Work out the finished part from the listing and answer in its coordinate system (mm). Face numbers are marked on the shaded views. A direction names the side the tool comes from. Round coordinates to 2 decimals unless told otherwise and drop trailing zeros. Loops run counter-clockwise (first coordinate to the right, second up) from the corner with the lowest first, then second, coordinate; pieces in that order, holes last. Notation, with made-up numbers: (-18, -5) - (7, -5) arc R10 ccw to (7, 7) - close; hole circle Ø2 at (50.5, 41). An arc over 180 degrees is marked (long way). Return JSON: item names as keys, results as strings.
from build123d import *

# Parameters (mm, degrees)
F1_DEPTH = 5
F2_R     = 1.65
F3_DEPTH = 2.001
F5_DEPTH = 5
F6_R     = 1


with BuildPart() as f1:
    # F0 (on Top) → F1 (new body)
    with BuildSketch(Plane.XY):
        Polygon((10, 5), (-10, 5), (-10, 0), (-15, 0), (-15, -2), (-10, -2), (10, -2), (15, -2), (15, 0), (10, 0), align=None)
    extrude(amount=F1_DEPTH)

    # F2 (on face) → F3 (cut, through all)
    with BuildSketch(Plane(origin=(0, 0, 0), x_dir=(-1, 0, 0), z_dir=(0, 1, 0))):
        with Locations((-12.5, 2.5)):
            Circle(F2_R)
        with Locations((12.5, 2.5)):
            Circle(F2_R)
    extrude(amount=-F3_DEPTH, mode=Mode.SUBTRACT)

    # F4 (on face) → F5 (cut, through all)
    with BuildSketch(Plane.XY.offset(5)):
        with BuildLine():
            Line((-9.5, -2), (-5.5, -2))
            ThreePointArc((-5.5, -2), (-7.5, 0), (-9.5, -2))
        make_face()
        with BuildLine():
            ThreePointArc((-0.5, -2), (-2.5, 0), (-4.5, -2))
            Line((-4.5, -2), (-0.5, -2))
        make_face()
        with BuildLine():
            ThreePointArc((4.5, -2), (2.5, 0), (0.5, -2))
            Line((0.5, -2), (4.5, -2))
        make_face()
        with BuildLine():
            ThreePointArc((9.5, -2), (7.5, 0), (5.5, -2))
            Line((5.5, -2), (9.5, -2))
        make_face()
        with BuildLine():
            ThreePointArc((-6.177124, 5), (-7.5, 5.5), (-8.822876, 5))
            Line((-8.822876, 5), (-6.177124, 5))
        make_face()
        with BuildLine():
            ThreePointArc((-1.177124, 5), (-2.5, 5.5), (-3.822876, 5))
            Line((-3.822876, 5), (-1.177124, 5))
        make_face()
        with BuildLine():
            Line((3.822876, 5), (1.177124, 5))
            ThreePointArc((1.177124, 5), (1.677124, 1.677124), (4.5, 3.5))
            ThreePointArc((4.5, 3.5), (4.322876, 4.322876), (3.822876, 5))
        make_face()
        with BuildLine():
            ThreePointArc((9.5, 3.5), (9.322876, 4.322876), (8.822876, 5))
            Line((8.822876, 5), (6.177124, 5))
            ThreePointArc((6.177124, 5), (6.677124, 1.677124), (9.5, 3.5))
        make_face()
        with BuildLine():
            Line((-6.177124, 5), (-8.822876, 5))
            ThreePointArc((-8.822876, 5), (-8.322876, 1.677124), (-5.5, 3.5))
            ThreePointArc((-5.5, 3.5), (-5.677124, 4.322876), (-6.177124, 5))
        make_face()
        with BuildLine():
            Line((-1.177124, 5), (-3.822876, 5))
            ThreePointArc((-3.822876, 5), (-3.322876, 1.677124), (-0.5, 3.5))
            ThreePointArc((-0.5, 3.5), (-0.677124, 4.322876), (-1.177124, 5))
        make_face()
        with BuildLine():
            ThreePointArc((3.822876, 5), (2.5, 5.5), (1.177124, 5))
            Line((1.177124, 5), (3.822876, 5))
        make_face()
        with BuildLine():
            Line((6.177124, 5), (8.822876, 5))
            ThreePointArc((8.822876, 5), (7.5, 5.5), (6.177124, 5))
        make_face()
    extrude(amount=-F5_DEPTH, mode=Mode.SUBTRACT)

    # F6
    f6_edges = [f1.edges().sort_by_distance(p)[0] for p in [
        (-10, 0, 2.5),
        (10, 0, 2.5),
        (10, 5, 2.5),
        (-10, 5, 2.5),
        (15, -1, 5),
        (15, -1, 0),
        (-15, -1, 0),
        (-15, -1, 5),
    ]]
    fillet(f6_edges, radius=F6_R)


solid = f1.part
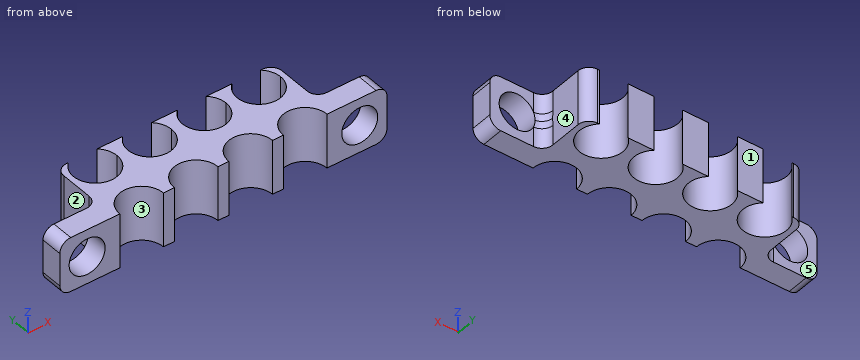
1) Section A-A (x = 12.5) is taken. Give the vertices of the cut face in (y, z).
Verdict:
{"outline": "(-2, 0) - (0, 0) - (0, 0.85) - (-2, 0.85) - close; (-2, 4.15) - (0, 4.15) - (0, 5) - (-2, 5) - close"}
2) Flat-ended cylindrical pins translate along their axes: pin 1 (1.5 mm diameter, centred on y = 2.5, z = 2.5, fed in from +X); pin 2 (2 mm diameter, centred on x = 8.5, z = 2.5, fed in from +Y); pin 3 (1 mm diameter, centred on x = 8, z = 1, fed in from +Y); pin 4 (2 mm diameter, centred on x = 13, z = 1.5, fed in from +Y). Find the tip coordinate at first contact, or state that the pin passes through.
Verdict:
{"pin 1": "stops at x = 10", "pin 2": "stops at y = 5", "pin 3": "stops at y = 1.77", "pin 4": "stops at y = 0"}
3) Section D-D (z = 3.7) is taken. Count the separate pieces of the cut face and the enclosed holes in it, and give its area (3 significant figures).
Verdict:
{"separate pieces": "3", "enclosed holes": "0", "area": "79.2 mm2"}
4) Find the intervals of material crossed by L1, parallel to Z at x = -12.5, y = -0.75; L2, parallel to X at y = 1.75, z = 3.25; L3, parallel to X at y = 3.5, z = 4.05, in increasing order.
Verdict:
{"L1": "z = 0 to 0.85, 4.15 to 5", "L2": "x = -10 to -8.47, -6.53 to -3.47, -1.53 to 1.53, 3.47 to 6.53, 8.47 to 10", "L3": "x = -10 to -9.5, -5.5 to -4.5, -0.5 to 0.5, 4.5 to 5.5, 9.5 to 10"}
5) Determine the mould class of the marked faces 3, 4 and 5 for opening direction X: pulls with the +X half, pulls with the -X half, needs draft (parallel to the pull), parting line crosses it, or undercut.
Verdict:
{"face 3": "undercut", "face 4": "pulls with the +X half", "face 5": "needs draft"}
6) Section C-C (x = 2.5) is taken. Give the vertices of the cut face in (y, z), and give its area (3 significant figures).
Verdict:
{"outline": "(0, 0) - (1.5, 0) - (1.5, 5) - (0, 5) - close", "area": "7.50 mm2"}
7) A tool of negligible diameter and unlimited length cuts with its end or side. For the marked faces 1 and 2, from which of +Z, -Z, +X, -X, +Y, -Y can it reach the whole face along a straight path? Write none if from no direction.
Verdict:
{"face 1": "+Z, -Z, +X, -X, +Y", "face 2": "+Z, -Z, -X, +Y"}
